Design review of the part built by this model. Coordinates are the model's own, in mm. Face numbers are marked on the shaded views. A direction names the side the tool comes from. Round coordinates to 2 decimals unless told otherwise and drop trailing zeros. Loops run counter-clockwise (first coordinate to the right, second up) from the corner with the lowest first, then second, coordinate; pieces in that order, holes last. Notation, with made-up numbers: (81, 34.25) - (103, 34.25) arc R15 ccw to (103, 47.25) - close; hole circle Ø9 at (28.5, -6). An arc over 180 degrees is marked (long way). Answer as CSV lines item,"result". Start each with the question number.
(1) Consider section A-A (y = 178). Give the boundary of the cut face in (x, z), and give its area (3 significant figures).
(2) For the marked faces 5 and 6, list the 3-axis set-ups (+Z, -Z, +X, -X, +Y, -Y) from which the entire face can be reached by the end or side of a thin tool; tool diameter is ignored.
(3) Consider section C-C (x = 50.5). Give the boundary of the cut face in (y, z), and give its area (3 significant figures).
(4) Mouldability with a two-part tool opening along X and no side actions: class the marked faces 1, 2, 3 and 4 as released by +X, released by -X, zero draft, split by the parting line, or undercut.
(5) For P1, Ø1.9, axis at x = 378, z = -455, coming from the -Y side; P2, Ø7.5, axis at x = 368.3, z = -416.56, coming from the +Y side, all flat-tipped, find the tip position at first contact; note any pin that passes through.
(6) Wall thickness on L1, parallel to X at y = 4, z = -416; L2, parallel to X at y = 1.75, z = -416.56 (3 decimals); L3, parallel to Z at x = 12.7, y = 2.75 (3 decimals): over which ranges is each line inside the solid? List them lowest first.
(7) Consider section B-B (z = -307). Give the boundary of the cut face in (x, y).
from build123d import *

# Parameters (mm, degrees)
SKETCH1_W            = 381
SKETCH1_H            = 429.26
BOSS_EXTRUDE1_DEPTH  = 6.35
SKETCH2_W            = 254
SKETCH2_H            = 203.2
CUT_EXTRUDE1_DEPTH   = 6.35
SKETCH3_W            = 381
SKETCH3_H            = 73.66
CUT_EXTRUDE2_DEPTH   = 6.35
SKETCH4_W            = 254
SKETCH4_H            = 6.35
CUT_EXTRUDE3_DEPTH   = 73.66
SKETCH6_W            = 6.35
SKETCH6_H            = 195.58
BOSS_EXTRUDE2_DEPTH  = 171.45
SKETCH7_W            = 6.35
SKETCH7_H            = 195.58
BOSS_EXTRUDE3_DEPTH  = 158.75
SKETCH8_W            = 6.35
SKETCH8_H            = 165.1
BOSS_EXTRUDE4_DEPTH  = 50.8
SKETCH9_W            = 6.35
SKETCH9_H            = 158.75
CUT_EXTRUDE4_DEPTH   = 50.8
SKETCH10_W           = 6.899940386
SKETCH10_H           = 177.8
BOSS_EXTRUDE5_DEPTH  = 50.8
SKETCH11_W           = 6.35
SKETCH11_H           = 171.45
CUT_EXTRUDE5_DEPTH   = 50.8
SKETCH13_W           = 0.549940386
SKETCH13_H           = 171.45
CUT_EXTRUDE6_DEPTH   = 50.8
SKETCH14_W           = 6.899940386
SKETCH14_H           = 177.8
CUT_EXTRUDE7_DEPTH   = 50.8
SKETCH15_W           = 6.35
SKETCH15_H           = 165.1
CUT_EXTRUDE8_DEPTH   = 50.8
SKETCH16_W           = 6.35
SKETCH16_H           = 144.78
BOSS_EXTRUDE6_DEPTH  = 25.4
SKETCH17_W           = 6.35
SKETCH17_H           = 144.78
BOSS_EXTRUDE7_DEPTH  = 19.05
SKETCH19_W           = 6.35
SKETCH19_H           = 139.7
BOSS_EXTRUDE8_DEPTH  = 50.8
SKETCH20_W           = 6.35
SKETCH20_H           = 195.58
BOSS_EXTRUDE9_DEPTH  = 31.75
SKETCH21_W           = 6.35
SKETCH21_H           = 139.7
BOSS_EXTRUDE10_DEPTH = 50.8
SKETCH22_W           = 6.35
SKETCH22_H           = 195.58
BOSS_EXTRUDE11_DEPTH = 50.8
SKETCH23_W           = 6.35
SKETCH23_H           = 50.8
BOSS_EXTRUDE12_DEPTH = 12.7
SKETCH24_W           = 6.35
SKETCH24_H           = 195.58
BOSS_EXTRUDE13_DEPTH = 12.7
SKETCH26_W           = 381
SKETCH26_H           = 210.82
CUT_EXTRUDE9_DEPTH   = 12.7
SKETCH27_R           = 3.175
CUT_EXTRUDE10_DEPTH  = 635
SKETCH28_R           = 3.175
CUT_EXTRUDE11_DEPTH  = 635


with BuildPart() as part:
    # Sketch1 → Boss-Extrude1 (new body)
    with BuildSketch(Plane(origin=(0, 0, 0), x_dir=(1, 0, 0), z_dir=(0, 1, 0))):
        with Locations((190.5, 214.63)):
            Rectangle(SKETCH1_W, SKETCH1_H)
    extrude(amount=BOSS_EXTRUDE1_DEPTH)

    # Sketch2 → Cut-Extrude1 (cut)
    with BuildSketch(Plane(origin=(0, 6.35, 0), x_dir=(1, 0, 0), z_dir=(0, 1, 0))):
        with Locations((190.5, 101.6)):
            Rectangle(SKETCH2_W, SKETCH2_H)
    extrude(amount=-CUT_EXTRUDE1_DEPTH, mode=Mode.SUBTRACT)

    # Sketch3 → Cut-Extrude2 (cut)
    with BuildSketch(Plane(origin=(0, 6.35, 0), x_dir=(1, 0, 0), z_dir=(0, 1, 0))):
        with Locations((190.5, 36.83)):
            Rectangle(SKETCH3_W, SKETCH3_H)
    extrude(amount=-CUT_EXTRUDE2_DEPTH, mode=Mode.SUBTRACT)

    # Sketch4 → Cut-Extrude3 (cut)
    with BuildSketch(Plane.XY.offset(-203.2)):
        with Locations((190.5, 3.175)):
            Rectangle(SKETCH4_W, SKETCH4_H)
    extrude(amount=-CUT_EXTRUDE3_DEPTH, mode=Mode.SUBTRACT)

    # Sketch6 → Boss-Extrude2 (add)
    with BuildSketch(Plane(origin=(0, 6.35, 0), x_dir=(1, 0, 0), z_dir=(0, 1, 0))):
        with Locations((377.825, 331.47)):
            Rectangle(SKETCH6_W, SKETCH6_H)
    extrude(amount=BOSS_EXTRUDE2_DEPTH)

    # Sketch7 → Boss-Extrude3 (add)
    with BuildSketch(Plane(origin=(0, 6.35, 0), x_dir=(1, 0, 0), z_dir=(0, 1, 0))):
        with Locations((3.175, 331.47)):
            Rectangle(SKETCH7_W, SKETCH7_H)
    extrude(amount=BOSS_EXTRUDE3_DEPTH)

    # Sketch8 → Boss-Extrude4 (add)
    with BuildSketch(Plane(origin=(0, 0, -429.26), x_dir=(-1, 0, 0), z_dir=(0, 0, -1))):
        with Locations((-3.175, 82.55)):
            Rectangle(SKETCH8_W, SKETCH8_H)
    extrude(amount=BOSS_EXTRUDE4_DEPTH)

    # Sketch9 → Cut-Extrude4 (cut)
    with BuildSketch(Plane.XY.offset(-233.68)):
        with Locations((3.175, 85.725)):
            Rectangle(SKETCH9_W, SKETCH9_H)
    extrude(amount=-CUT_EXTRUDE4_DEPTH, mode=Mode.SUBTRACT)

    # Sketch10 → Boss-Extrude5 (add)
    with BuildSketch(Plane(origin=(0, 0, -429.26), x_dir=(-1, 0, 0), z_dir=(0, 0, -1))):
        with Locations((-377.550029807, 88.9)):
            Rectangle(SKETCH10_W, SKETCH10_H)
    extrude(amount=BOSS_EXTRUDE5_DEPTH)

    # Sketch11 → Cut-Extrude5 (cut)
    with BuildSketch(Plane.XY.offset(-233.68)):
        with Locations((377.825, 92.075)):
            Rectangle(SKETCH11_W, SKETCH11_H)
    extrude(amount=-CUT_EXTRUDE5_DEPTH, mode=Mode.SUBTRACT)

    # Sketch13 → Cut-Extrude6 (cut)
    with BuildSketch(Plane.XY.offset(-429.26)):
        with Locations((374.375029807, 92.075)):
            Rectangle(SKETCH13_W, SKETCH13_H)
    extrude(amount=-CUT_EXTRUDE6_DEPTH, mode=Mode.SUBTRACT)

    # Sketch14 → Cut-Extrude7 (cut)
    with BuildSketch(Plane(origin=(0, 0, -480.06), x_dir=(-1, 0, 0), z_dir=(0, 0, -1))):
        with Locations((-377.550029807, 88.9)):
            Rectangle(SKETCH14_W, SKETCH14_H)
    extrude(amount=-CUT_EXTRUDE7_DEPTH, mode=Mode.SUBTRACT)

    # Sketch15 → Cut-Extrude8 (cut)
    with BuildSketch(Plane(origin=(0, 0, -480.06), x_dir=(-1, 0, 0), z_dir=(0, 0, -1))):
        with Locations((-3.175, 82.55)):
            Rectangle(SKETCH15_W, SKETCH15_H)
    extrude(amount=-CUT_EXTRUDE8_DEPTH, mode=Mode.SUBTRACT)

    # Sketch16 → Boss-Extrude6 (add)
    with BuildSketch(Plane(origin=(0, 177.8, 0), x_dir=(1, 0, 0), z_dir=(0, 1, 0))):
        with Locations((377.825, 356.87)):
            Rectangle(SKETCH16_W, SKETCH16_H)
    extrude(amount=BOSS_EXTRUDE6_DEPTH)

    # Sketch17 → Boss-Extrude7 (add)
    with BuildSketch(Plane(origin=(0, 165.1, 0), x_dir=(1, 0, 0), z_dir=(0, 1, 0))):
        with Locations((3.175, 356.87)):
            Rectangle(SKETCH17_W, SKETCH17_H)
    extrude(amount=-BOSS_EXTRUDE7_DEPTH)

    # Sketch19 → Boss-Extrude8 (add)
    with BuildSketch(Plane(origin=(0, 0, -429.26), x_dir=(-1, 0, 0), z_dir=(0, 0, -1))):
        with Locations((-3.175, 120.65)):
            Rectangle(SKETCH19_W, SKETCH19_H)
    extrude(amount=BOSS_EXTRUDE8_DEPTH)

    # Sketch20 → Boss-Extrude9 (add)
    with BuildSketch(Plane(origin=(0, 190.5, 0), x_dir=(1, 0, 0), z_dir=(0, 1, 0))):
        with Locations((3.175, 382.27)):
            Rectangle(SKETCH20_W, SKETCH20_H)
    extrude(amount=-BOSS_EXTRUDE9_DEPTH)

    # Sketch21 → Boss-Extrude10 (add)
    with BuildSketch(Plane(origin=(0, 0, -429.26), x_dir=(-1, 0, 0), z_dir=(0, 0, -1))):
        with Locations((-377.825, 133.35)):
            Rectangle(SKETCH21_W, SKETCH21_H)
    extrude(amount=BOSS_EXTRUDE10_DEPTH)

    # Sketch22 → Boss-Extrude11 (add)
    with BuildSketch(Plane(origin=(0, 203.2, 0), x_dir=(1, 0, 0), z_dir=(0, 1, 0))):
        with Locations((377.825, 382.27)):
            Rectangle(SKETCH22_W, SKETCH22_H)
    extrude(amount=-BOSS_EXTRUDE11_DEPTH)

    # Sketch23 → Boss-Extrude12 (add)
    with BuildSketch(Plane.XZ.offset(-63.5)):
        with Locations((377.825, -454.66)):
            Rectangle(SKETCH23_W, SKETCH23_H)
    extrude(amount=BOSS_EXTRUDE12_DEPTH)

    # Sketch24 → Boss-Extrude13 (add)
    with BuildSketch(Plane(origin=(0, 190.5, 0), x_dir=(1, 0, 0), z_dir=(0, 1, 0))):
        with Locations((3.175, 382.27)):
            Rectangle(SKETCH24_W, SKETCH24_H)
    extrude(amount=BOSS_EXTRUDE13_DEPTH)

    # Sketch26 → Cut-Extrude9 (cut)
    with BuildSketch(Plane(origin=(0, 6.35, 0), x_dir=(1, 0, 0), z_dir=(0, 1, 0))):
        with Locations((190.5, 179.07)):
            Rectangle(SKETCH26_W, SKETCH26_H)
    extrude(amount=-CUT_EXTRUDE9_DEPTH, mode=Mode.SUBTRACT)

    # Sketch27 → Cut-Extrude10 (cut)
    with BuildSketch(Plane(origin=(0, 6.35, 0), x_dir=(1, 0, 0), z_dir=(0, 1, 0))):
        with Locations((368.3, 416.56)):
            Circle(SKETCH27_R)
    extrude(amount=-CUT_EXTRUDE10_DEPTH, mode=Mode.SUBTRACT)

    # Sketch28 → Cut-Extrude11 (cut)
    with BuildSketch(Plane(origin=(0, 6.35, 0), x_dir=(1, 0, 0), z_dir=(0, 1, 0))):
        with Locations((12.7, 416.56)):
            Circle(SKETCH28_R)
    extrude(amount=-CUT_EXTRUDE11_DEPTH, mode=Mode.SUBTRACT)


solid = part.part
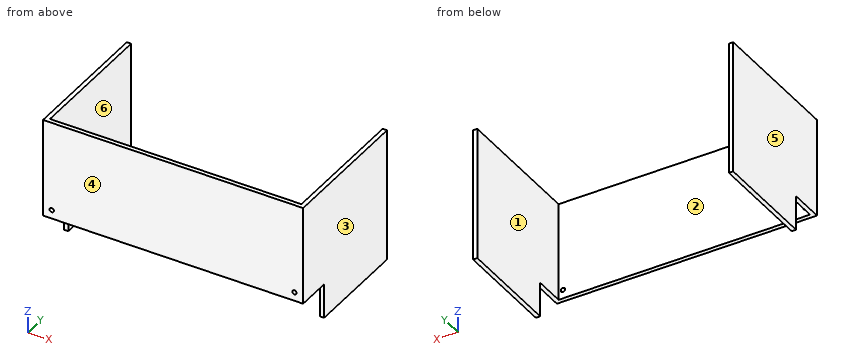
Determined:
1,outline,"(0, -480.06) - (6.35, -480.06) - (6.35, -284.48) - (0, -284.48) - close; (374.65, -480.06) - (381, -480.06) - (381, -284.48) - (374.65, -284.48) - close"
1,area,"2,480 mm^2"
2,face 5,"+Z, -Z, -X, +Y, -Y"
2,face 6,"+Z, -Z, +Y"
3,outline,"(0, -429.26) - (6.35, -429.26) - (6.35, -284.48) - (0, -284.48) - close"
3,area,"919 mm^2"
4,face 1,"undercut"
4,face 2,"undercut"
4,face 3,"released by +X"
4,face 4,"zero draft"
5,P1,"stops at y = 50.8"
5,P2,"stops at y = 6.35"
6,L1,"x = 0 to 9.57, 15.83 to 365.17, 371.43 to 381"
6,L2,"x = 0 to 9.525, 15.875 to 365.125, 371.475 to 381"
6,L3,"z = -429.26 to -419.735, -413.385 to -284.48"
7,outline,"(0, 0) - (381, 0) - (381, 203.2) - (374.65, 203.2) - (374.65, 6.35) - (6.35, 6.35) - (6.35, 203.2) - (0, 203.2) - close"
